Build history of the part. All positions in model axes, mm. Face numbers are marked on the shaded views. Coordinates: 2 decimals unless noted, no trailing zeros. Loops run counter-clockwise (first coordinate to the right, second up) from the corner with the lowest first, then second, coordinate; pieces in that order, holes last. Notation, with made-up numbers: (-21, -0.5) - (33, -0.5) arc R36 ccw to (33, 38.5) - close; hole circle Ø3 at (-32, 44.25). An arc over 180 degrees is marked (long way). One line per item, written item: value.
Autodesk Inventor part; units mm, degrees
ref_plane "YZ Plane" through (0, 0, 0) normal (1, 0, 0) x (0, 1, 0)
ref_plane "XZ Plane" through (0, 0, 0) normal (0, 1, 0) x (-1, 0, 0)
ref_plane "XY Plane" through (0, 0, 0) normal (0, 0, 1) x (1, 0, 0)
sketch "Szkic1" plane through (0, 0, 0) normal (0, 0, 1) x (1, 0, 0)
  line L0 (200, -100) -> (-200, -100)
  line L1 (-200, -100) -> (-200, 100)
  line L2 (-200, 100) -> (200, 100)
  line L3 (200, 100) -> (200, -100)
  line L4 (200, -100) -> (-200, 100) construction
  line L5 (-200, -100) -> (200, 100) construction
  point P0 (0, 0)
  dimension "d0" = 400
  dimension "d1" = 200
extrude "Wyciągnięcie proste1" add sketch "Szkic1" along normal mid plane 6
sketch "Szkic2" plane through (0, 0, 3) normal (0, 0, 1) x (1, 0, 0)
  line L0 (-200, -100) -> (200, -100)
  line L1 (20, -100) -> (100, -100)
  line L2 (100, -100) -> (100, 60)
  line L3 (100, 60) -> (20, 60)
  line L4 (20, 60) -> (20, -100)
  line L5 (200, -100) -> (200, 100)
  line L6 (-22, 11) -> (-10, 11)
  line L7 (-10, 11) -> (-10, -5)
  line L8 (-10, -5) -> (-22, -5)
  line L9 (-22, -5) -> (-22, 11)
  line L10 (-71, -29) -> (-10, -29)
  line L11 (-10, -29) -> (-10, -70)
  line L12 (-10, -70) -> (-71, -70)
  line L13 (-71, -70) -> (-71, -29)
  point P0 (0, 0)
  point P1 (-10, 3)
  dimension "d4" = 80
  dimension "d5" = 160
  dimension "d6" = 100
  dimension "d7" = 16
  dimension "d8" = 12
  dimension "d9" = 95
  dimension "d10" = 61
  dimension "d11" = 41
  dimension "d12" = 30
  dimension "d13" = 30
  dimension "d14" = 30
extrude "Wyciągnięcie proste2" cut sketch "Szkic2" against normal through all contours L4 L3 L2 L0
sketch "Szkic3" plane through (0, 0, -3) normal (0, 0, -1) x (-1, 0, 0)
  line L0 (71, -29) -> (10, -29)
  line L1 (71, -70) -> (71, -29)
  line L2 (10, -70) -> (71, -70)
  line L3 (10, -29) -> (10, -70)
  line L4 (10, -5) -> (22, -5)
  line L5 (22, -5) -> (22, 11)
  line L6 (22, 11) -> (10, 11)
  line L7 (10, 11) -> (10, -5)
  point P0 (0, 0)
  point P1 (10, 3)
extrude "Wyciągnięcie proste3" cut sketch "Szkic3" against normal blind 5 contours L7 L6 L5 L4
sketch "Szkic4" plane through (0, 0, -3) normal (0, 0, -1) x (-1, 0, 0)
  line L0 (71, -29) -> (10, -29)
  line L1 (71, -70) -> (71, -29)
  line L2 (10, -70) -> (71, -70)
  line L3 (10, -29) -> (10, -70)
  point P0 (0, 0)
extrude "Wyciągnięcie proste4" cut sketch "Szkic4" against normal blind 3
sketch "Szkic6" plane through (0, 0, -3) normal (0, 0, -1) x (-1, 0, 0)
  line L0 (22, -5) -> (10, -5)
  line L1 (12, -5) -> (12, -21)
  line L2 (12, -21) -> (82, -21)
  line L3 (82, -21) -> (82, -40)
  line L4 (82, -40) -> (71, -40)
  line L5 (71, -29) -> (71, -70)
  line L6 (71, -60) -> (82, -60)
  line L7 (71, -70) -> (10, -70)
  line L8 (10, -70) -> (10, -29)
  line L9 (10, -29) -> (71, -29)
  line L10 (71, -29) -> (71, -70)
  line L11 (10, 11) -> (22, 11)
  line L12 (22, 11) -> (22, -5)
  line L13 (22, -5) -> (10, -5)
  line L14 (10, -5) -> (10, 11)
  line L15 (-20, 60) -> (-20, -100)
  line L16 (-20, -100) -> (200, -100)
  line L17 (200, -100) -> (200, 100)
  line L18 (200, 100) -> (-200, 100)
  line L19 (-200, 100) -> (-200, -100)
  line L20 (-200, -100) -> (-100, -100)
  line L21 (-100, -100) -> (-100, 60)
  line L22 (-100, 60) -> (-20, 60)
  line L23 (82, -60) -> (82, -100)
  line L24 (-20, -100) -> (200, -100)
  line L25 (20, -5) -> (20, -13)
  line L26 (20, -13) -> (90, -13)
  line L27 (90, -13) -> (90, -100)
  point P0 (0, 0)
  point P1 (12, -13)
  dimension "d21" = 8
  dimension "d22" = 32
  dimension "d23" = 8
  dimension "d24" = 8
  dimension "d25" = 20
  dimension "d26" = 40
  dimension "d27" = 8
  dimension "d28" = 8
extrude "Wyciągnięcie proste5" cut sketch "Szkic6" against normal blind 3 contours L25 L26 L27 L16 L23 L6 L5 L4 L3 L2 L1 L0
sketch "Szkic7" plane through (0, 0, 3) normal (0, 0, 1) x (1, 0, 0)
  line L0 (-200, 100) -> (200, 100)
  line L1 (200, 100) -> (200, -100)
  line L2 (-200, 100) -> (200, 100)
  line L3 (200, 100) -> (200, 92)
  line L4 (200, 92) -> (-200, 92)
  line L5 (-200, 92) -> (-200, 100)
  point P0 (0, 0)
  dimension "d31" = 8
extrude "Wyciągnięcie proste6" add sketch "Szkic7" along normal blind 15
sketch "Szkic8" plane through (-200, 92, 3) normal (0, -1, 0) x (1, 0, 0)
  line L0 (400, 15) -> (400, -6)
  line L1 (0, -6) -> (0, 15)
  line L2 (400, 13) -> (0, 13)
  line L3 (0, 13) -> (0, 2)
  line L4 (0, 2) -> (400, 2)
  line L5 (400, 2) -> (400, 13)
  line L6 (0, 15) -> (400, 15)
  point P0 (200, -3)
  point P1 (0, 13)
  dimension "d34" = 11
  dimension "d35" = 2
extrude "Wyciągnięcie proste7" cut sketch "Szkic8" against normal blind 3 contours L0 L4 L1 L2
sketch "Szkic9" plane through (0, 0, -3) normal (0, 0, -1) x (-1, 0, 0)
  line L0 (156, 85) -> (170, 85)
  line L1 (170, 85) -> (170, 55)
  line L2 (170, 55) -> (156, 55)
  line L3 (156, 55) -> (156, 85)
  line L4 (200, -100) -> (200, 100)
  line L5 (200, 100) -> (-200, 100)
  circle A0 centre (163, 78) radius 6
  line L6 (90, -100) -> (200, -100)
  line L7 (159, 55) -> (159, -100)
  line L8 (167, 55) -> (167, -100)
  point P0 (0, 0)
  point P1 (163, 55)
  dimension "d38" = 14
  dimension "d39" = 30
  dimension "d40" = 30
  dimension "d41" = 15
  dimension "d42" = 12
  dimension "d43" = 23
  dimension "d44" = 7
  dimension "d49" = 8
  dimension "d50" = 33
extrude "Wyciągnięcie proste8" cut sketch "Szkic9" against normal blind 6 contours A0
extrude "Wyciągnięcie proste9" cut sketch "Szkic9" against normal blind 3 contours L0 L1 L2 L3
extrude "Wyciągnięcie proste10" cut sketch "Szkic9" against normal blind 3 contours L2 L8 L6 L7
properties part number "FrontWall"
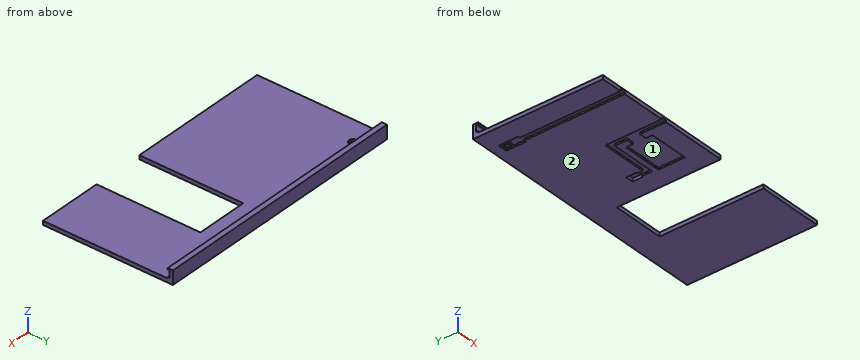
Item 1: Pull direction Y, two halves, no side cores. Call the marked faces 1 and 2: released by +Y, released by -Y, zero draft, split by the parting line, or undercut.
Check result:
face 1: undercut
face 2: zero draft
Item 2: Cut at A-A, the plane y = 78. Write the cut outline in (x, z).
Check result:
outline: (-200, -3) - (-170, -3) - (-170, 0) - (-169, 0) - (-169, 3) - (-200, 3) - close; (-157, 0) - (-156, 0) - (-156, -3) - (200, -3) - (200, 3) - (-157, 3) - close
Item 3: Cut at D-D, the plane y = -46. Write the cut outline in (x, z), then the cut area to 3 significant figures.
Check result:
outline: (-200, -3) - (-167, -3) - (-167, 0) - (-159, 0) - (-159, -3) - (-90, -3) - (-90, 0) - (-10, 0) - (-10, -3) - (20, -3) - (20, 3) - (-200, 3) - close; (100, -3) - (200, -3) - (200, 3) - (100, 3) - close
area: 1,660 mm^2
Item 4: Cut at C-C, the plane x = -163. Write the cut outline in (y, z), then the cut area to 3 significant figures.
Check result:
outline: (-100, 0) - (72, 0) - (72, 3) - (-100, 3) - close; (84, 0) - (85, 0) - (85, -3) - (100, -3) - (100, 18) - (92, 18) - (92, 16) - (95, 16) - (95, 5) - (92, 5) - (92, 3) - (84, 3) - close
area: 696 mm^2
Item 5: Drop flat-ended pins along their axis: P1, Ø1, axis at x = -4, z = 17, coming from the -Y side; P2, Ø2, axis at x = -34.5, y = 2.5, coming from the +Z side; P3, Ø1, axis at x = 108, z = 14, coming from the -Y side. Give the stop position or say it passes through.
Check result:
P1: stops at y = 92
P2: stops at z = 3
P3: stops at y = 95
Item 6: Cut at B-B, the plane x = -57. Write the cut outline in (y, z), then the cut area to 3 significant figures.
Check result:
outline: (-100, -3) - (-70, -3) - (-70, 0) - (-29, 0) - (-29, -3) - (-21, -3) - (-21, 0) - (-13, 0) - (-13, -3) - (100, -3) - (100, 18) - (92, 18) - (92, 16) - (95, 16) - (95, 5) - (92, 5) - (92, 3) - (-100, 3) - close
area: 1,140 mm^2
Item 7: Probe probe 1 along Y at (x, z) = (-26, -2); probe 2 along Y at (x, z) = (-163, 1.65); probe 3 along X at (y, z) = (77, -1.5). List the from-to ranges inside material, lowest first. Write a range as from..to.
Check result:
probe 1: y = -100..-70, -29..-21, -13..100
probe 2: y = -100..72, 84..100
probe 3: x = -200..-170, -156..200
